Model file for the job. Use its own axes, mm. Face numbers are marked on the shaded views. Round coordinates to 2 decimals unless told otherwise and drop trailing zeros. Loops run counter-clockwise (first coordinate to the right, second up) from the corner with the lowest first, then second, coordinate; pieces in that order, holes last.
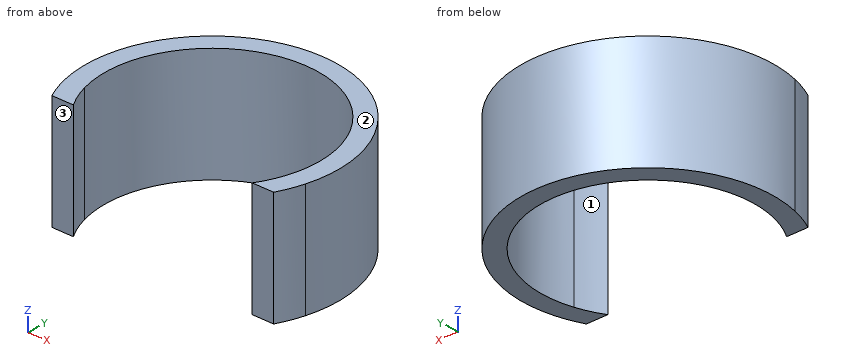
from build123d import *

# Parameters (mm, degrees)
F1_DEPTH = 15


with BuildPart() as f1:
    # F0 (on Top) → F1 (new body)
    with BuildSketch(Plane.XY):
        with BuildLine():
            ThreePointArc((-13.416408, -4), (0, 14), (13.416408, -4))
            ThreePointArc((13.416408, -4), (12.774857, -5.727392), (11.911998, -7.355563))
            Line((11.911998, -7.355563), (14.769756, -7.355563))
            ThreePointArc((14.769756, -7.355563), (15.479974, -5.711427), (16.007811, -4))
            ThreePointArc((16.007811, -4), (0, 16.5), (-16.007811, -4))
            ThreePointArc((-16.007811, -4), (-15.479974, -5.711427), (-14.769756, -7.355563))
            Line((-14.769756, -7.355563), (-11.911998, -7.355563))
            ThreePointArc((-11.911998, -7.355563), (-12.774857, -5.727392), (-13.416408, -4))
        make_face()
    extrude(amount=F1_DEPTH)


solid = f1.part
Q1. Flat gauge pins, fed straight in: P1, Ø6, axis at x = 11, z = 5.5, coming from the -Y side; P2, Ø1, axis at y = -3, z = 6.5, coming from the -X side; P3, Ø5, axis at x = -7.5, z = 4, coming from the +Y side. Where does each tip first touch, or does it go through?
Q2. Slice it at B-B on y = -3.25. Give the cut face in (x, z).
Q3. Pull direction Y, two halves, no side cores. Call the marked faces 1, 2 and 3: pulls with the +Y half, pulls with the -Y half, needs draft (parallel to the pull), parting line crosses it, or undercut.
Q4. Slice it at D-D on x = 0. Give the cut face in (y, z).
Q5. Probe line 1 (X direction, y = 0, z = 10); line 2 (X direction, y = 6, z = 8.75); line 3 (Y direction, x = -4, z = 5.5). List the from-to ranges inside material, lowest first.
Q6. Slice it at C-C on z = 13.5. Give the cut face in (x, y).
Q7. Slice it at A-A on x = 13. Give the cut face in (y, z), plus the area to 3 significant figures.
Reply:
1. P1: stops at y = -7.36
1. P2: stops at x = -16.31
1. P3: stops at y = 15.72
2. outline: (-16.18, 0) - (-13.62, 0) - (-13.62, 15) - (-16.18, 15) - close; (13.62, 0) - (16.18, 0) - (16.18, 15) - (13.62, 15) - close
3. face 1: undercut
3. face 2: needs draft
3. face 3: pulls with the -Y half
4. outline: (14, 0) - (16.5, 0) - (16.5, 15) - (14, 15) - close
5. line 1: x = -16.5 to -14, 14 to 16.5
5. line 2: x = -15.37 to -12.65, 12.65 to 15.37
5. line 3: y = 13.42 to 16.01
6. outline: (-16.01, -4) arc R16.5 ccw to (-14.77, -7.36) - (-11.91, -7.36) arc R14 cw to (-13.42, -4) arc R14 cw (long way) to (13.42, -4) arc R14 cw to (11.91, -7.36) - (14.77, -7.36) arc R16.5 ccw to (16.01, -4) arc R16.5 ccw (long way) to start
7. outline: (-7.36, 0) - (-5.2, 0) - (-5.2, 15) - (-7.36, 15) - close; (5.2, 0) - (10.16, 0) - (10.16, 15) - (5.2, 15) - close
7. area: 107 mm2
